```python
from build123d import *

# Parameters (mm, degrees)
F1_DEPTH = 40
F2_DEPTH = 5
F3_SIZE  = 5


with BuildPart() as f1:
    # F0 (on Top) → F1 (new body)
    with BuildSketch(Plane.XY):
        Polygon((-17.5, 7.248737), (-17.5, -7.248737), (-7.248737, -17.5), (7.248737, -17.5), (17.5, -7.248737), (17.5, 7.248737), (7.248737, 17.5), (-7.248737, 17.5), align=None)
        Polygon((-6.213203, -15), (-15, -6.213203), (-15, 6.213203), (-6.213203, 15), (6.213203, 15), (15, 6.213203), (15, -6.213203), (6.213203, -15), align=None, mode=Mode.SUBTRACT)
    extrude(amount=F1_DEPTH)

    # F0 (on Top) → F2 (join)
    with BuildSketch(Plane.XY):
        Polygon((-15, 6.213203), (-15, -6.213203), (-6.213203, -15), (6.213203, -15), (15, -6.213203), (15, 6.213203), (6.213203, 15), (-6.213203, 15), align=None)
    extrude(amount=F2_DEPTH)

    # F3
    f3_edges = [f1.edges().sort_by_distance(p)[0] for p in [
        (12.374369, -12.374369, 0),
        (0, -17.5, 0),
        (17.5, 0, 0),
        (12.374369, 12.374369, 0),
        (0, 17.5, 0),
        (-12.374369, 12.374369, 0),
        (-17.5, 0, 0),
        (-12.374369, -12.374369, 0),
    ]]
    chamfer(f3_edges, length=F3_SIZE)


solid = f1.part
```
Geometry: final body of the model. Coordinates: model frame, mm. A direction names the side the tool comes from. Round coordinates to 2 decimals unless told otherwise and drop trailing zeros. Loops run counter-clockwise (first coordinate to the right, second up) from the corner with the lowest first, then second, coordinate; pieces in that order, holes last.
Item 1: Section B-B, the plane y = 4. Output: boundary loops of the cut face in (x, z).
Checked values:
outline: (-17.5, 5) - (-12.5, 0) - (12.5, 0) - (17.5, 5) - (17.5, 40) - (15, 40) - (15, 5) - (-15, 5) - (-15, 40) - (-17.5, 40) - close
Item 2: Line query: L1, parallel to Y at x = -4.5, z = 6; L2, parallel to Z at x = 6, y = 6.5. Output: solid intervals per line, ascending.
Checked values:
L1: y = -17.5 to -15, 15 to 17.5
L2: z = 0 to 5
Item 3: Section D-D, the plane z = 3. Output: boundary loops of the cut face in (x, y).
Checked values:
outline: (-15.5, -6.42) - (-6.42, -15.5) - (6.42, -15.5) - (15.5, -6.42) - (15.5, 6.42) - (6.42, 15.5) - (-6.42, 15.5) - (-15.5, 6.42) - close
Item 4: Mould query, pull axis X, two halves, no side actions, for faces 1 (the flat face through (15, 0, 22)), 2 (the flat face through (15, -0.1, 2.5)), 3 (the flat face through (0, 0, 0)). Classes: released by +X, released by -X, zero draft, split by the parting line, or undercut.
Checked values:
face 1: undercut
face 2: released by +X
face 3: zero draft
Item 5: Section A-A, the plane z = 25. Output: boundary loops of the cut face in (x, y).
Checked values:
outline: (-17.5, -7.25) - (-7.25, -17.5) - (7.25, -17.5) - (17.5, -7.25) - (17.5, 7.25) - (7.25, 17.5) - (-7.25, 17.5) - (-17.5, 7.25) - close; hole (-15, -6.21) - (-6.21, -15) - (6.21, -15) - (15, -6.21) - (15, 6.21) - (6.21, 15) - (-6.21, 15) - (-15, 6.21) - close
Item 6: Reachability of faces 4 (the flat face through (0, -17.5, 22)), 5 (the flat face through (10.545, 10.668, 22.255)) from +Z, -Z, +X, -X, +Y, -Y: full face, straight path, thin tool, end or side. Return the list, or none.
Checked values:
face 4: +Z, -Z, +X, -X, -Y
face 5: +Z
Item 7: Contact query for flat-ended pins moving along their axis: P1, Ø10, axis at y = -12.5, z = 34.5, coming from the -X side; P2, Ø1, axis at x = -6.5, y = -12, coming from the +Z side; P3, Ø2, axis at x = -14, z = 34, coming from the +Y side. Output: stop coordinate, or through.
Checked values:
P1: stops at x = -17.25
P2: stops at z = 5
P3: stops at y = 11.75
